Autodesk Inventor part; units mm, degrees
ref_plane "YZ Plane" through (0, 0, 0) normal (1, 0, 0) x (0, 1, 0)
ref_plane "XZ Plane" through (0, 0, 0) normal (0, 1, 0) x (-1, 0, 0)
ref_plane "XY Plane" through (0, 0, 0) normal (0, 0, 1) x (1, 0, 0)
sketch "Sketch2" plane through (0, 0, 0) normal (1, 0, 0) x (0, 1, 0)
  line L0 (40, 12.5) -> (40, -12.5)
  line L1 (40, -12.5) -> (-40, -12.5)
  line L2 (-40, -12.5) -> (-40, 12.5)
  line L3 (-40, 12.5) -> (40, 12.5)
  point P0 (0, 0)
  dimension "d11" = 25
  dimension "d12" = 80
  dimension "d13" = 40
  dimension "d14" = 12.5
extrude "Extrusion2" add sketch "Sketch2" along normal blind 38
full round fillet "Full Round Fillet1" first side at (25.3333, 13.3333, 12.5) centre faces at (12.6667, 40, -4.1667) second side at (25.3333, -13.3333, -12.5)
full round fillet "Full Round Fillet2" first side at (25.3333, 5.0001, 12.5) centre faces at (12.6667, -40, 4.1667) second side at (25.3333, -17.5, -12.5)
sketch "Sketch3" plane through (38, 27.5, -12.5) normal (0, 0, -1) x (-1, 0, 0)
  circle A0 centre (21, -27.5) radius 10
  line L0 (38, -55) -> (38, 0)
  point P0 (38, -27.5)
  point P1 (38, -27.5)
  dimension "d15" = 20
  dimension "d16" = 17
sketch "Sketch4" plane through (38, 0, 0) normal (1, 0, 0) x (0, 0, -1)
  circle A0 centre (0, -20) radius 6
  circle A1 centre (0, 20) radius 6
  point P0 (0, 0)
  dimension "d17" = 12
  dimension "d18" = 12
  dimension "d31" = 40
  dimension "d32" = 20
extrude "Extrusion3" cut sketch "Sketch3" against normal blind 42
extrude "Extrusion4" cut sketch "Sketch4" against normal blind 42
thread "Thread4"
thread "Thread7"
thread "Thread8"
properties part number "Junção Fuso" material "Steel AISI 4142 380 QT"
The listing builds one solid part. Answer for the finished solid, in the listing's coordinates (mm). Give positions to 0.01 mm unless a question says otherwise; leave off trailing zeros. Order: outer loops, then holes, each group sorted by start corner. A loop starts at its lowest first (then second) coordinate and runs counter-clockwise, first axis right, second up. Notation, with made-up numbers: (-14, 41.5) -> (5, 41.5) arc R18 ccw to (5, 72.5) -> close; hole circle Ø4 at (32, 20.5). An arc over 180 degrees is marked (long way). Write each question's results on one line, items separated by ' | '.
Q1. Determine the mould class of faces 1 (the face through (7.46, 3, -0.18)), 2 (the face through (19.266, -36.241, 8.936)), 3 (the face through (19.27, -14.05, 0.78)), 4 (the face through (27.2, 0.4, -12.5)) for opening direction Z: pulls with the +Z half, pulls with the -Z half, needs draft (parallel to the pull), parting line crosses it, or undercut.
Checked values:
face 1: needs draft | face 2: pulls with the +Z half | face 3: undercut | face 4: pulls with the -Z half
Q2. The part is cut by section A-A, the plane x = 17. State how many separate pieces and enclosed holes the cut face has, and give its area (3 significant figures).
Checked values:
separate pieces: 2 | enclosed holes: 2 | area: 1,140 mm^2
Q3. The part is cut by section C-C, the plane y = -20. Give the vertices of the cut face in (x, z).
Checked values:
outline: (0, -12.5) -> (38, -12.5) -> (38, -6) -> (0, -6) -> close; (0, 6) -> (38, 6) -> (38, 12.5) -> (0, 12.5) -> close
Q4. Straight lines are drawn through the part: probe 1 along Y at (x, z) = (17, -1); probe 2 along Y at (x, z) = (3, 1.5); probe 3 along Y at (x, z) = (31, 2.25). For each, find the intervals that lie inside material, in ascending order. Write a range as from..to.
Checked values:
probe 1: y = -39.96..-25.92, -14.08..-10, 10..14.08, 25.92..39.96 | probe 2: y = -39.91..-25.81, -14.19..14.19, 25.81..39.91 | probe 3: y = -39.8..-25.56, -14.44..14.44, 25.56..39.8
Q5. The part is cut by section B-B, the plane z = -4. Give the vertices of the cut face in (x, y).
Checked values:
outline: (0, -39.34) -> (38, -39.34) -> (38, -24.47) -> (0, -24.47) -> close; (0, -15.53) -> (38, -15.53) -> (38, 15.53) -> (0, 15.53) -> close; (0, 24.47) -> (38, 24.47) -> (38, 39.34) -> (0, 39.34) -> close; hole circle Ø20 at (17, 0)
Q6. This flat-tipped pin is pushed along its axis until it touches: P1, Ø1.5, axis at x = 16, z = -5.5, coming from the +Y side. Where does it stop, or does it pass through?
Checked values:
P1: stops at y = 39.06
Q7. The part is cut by section D-D, the plane y = 0. Give the vertices of the cut face in (x, z), and give its area (3 significant figures).
Checked values:
outline: (0, -12.5) -> (7, -12.5) -> (7, 12.5) -> (0, 12.5) -> close; (27, -12.5) -> (38, -12.5) -> (38, 12.5) -> (27, 12.5) -> close | area: 450 mm^2
